Design review of the part shown in the three views and the two pictorial views. Dimensions are in mm from the part's minimum x, y and z. A direction names the side the tool comes from. Round coordinates to 2 decimals unless told otherwise and drop trailing zeros. Loops run counter-clockwise (first coordinate to the right, second up) from the corner with the lowest first, then second, coordinate; pieces in that order, holes last. Notation, with made-up numbers: M 0,-25.75 L 27,-25.75 A16 ccw 27,-6.75 Z; hole C -36,-34 d7. An arc over 180 degrees is marked long. Return JSON: item names as keys, results as strings. Group by question number.
Q1. Consider section D-D (x = 104.5). State the section outline as (y, z) points.
Q2. Consider section B-B (y = 57.15). State the section outline as (x, z) points, and give its area (3 significant figures).
Q3. To check wall thickness, follow line 1 along Y through (x, z) = (57.15, 96.75); line 2 along Z through (x, y) = (24, 40.5). State the ranges of each line that lie inside material, in increasing order.
Q4. Clearance check with flat-ended pins moving along their axes: pin 1 Ø2.5 at (y, z) = (4.5, 4) entering from +X (1 decimal); pin 2 Ø2 at (x, z) = (29, 87.5) entering from -Y; pin 3 Ø5.5 at (x, y) = (57.5, 5) entering from -Z; pin 4 Ø1.5 at (x, y) = (95, 102) entering from -Z. State where each tip first meets the part, or that it passes through.
Q5. Draft analysis for pull direction X (two halves, no side actions). For the marked faces 1 and 2, state which applies: pulls with the +X half, pulls with the -X half, needs draft (parallel to the pull), parting line crosses it, or undercut.
Q6. Consider section A-A (x = 57.15). State the section outline as (y, z) points, and give its area (3 significant figures).
Q7. Consider section C-C (z = 28.5). State the section outline as (x, y) points.
Q8. For the marked faces 3, 4 and 5, list the 3-axis set-ups (+Z, -Z, +X, -X, +Y, -Y) from which the entire face can be reached by the end or side of a thin tool; tool diameter is ignored.
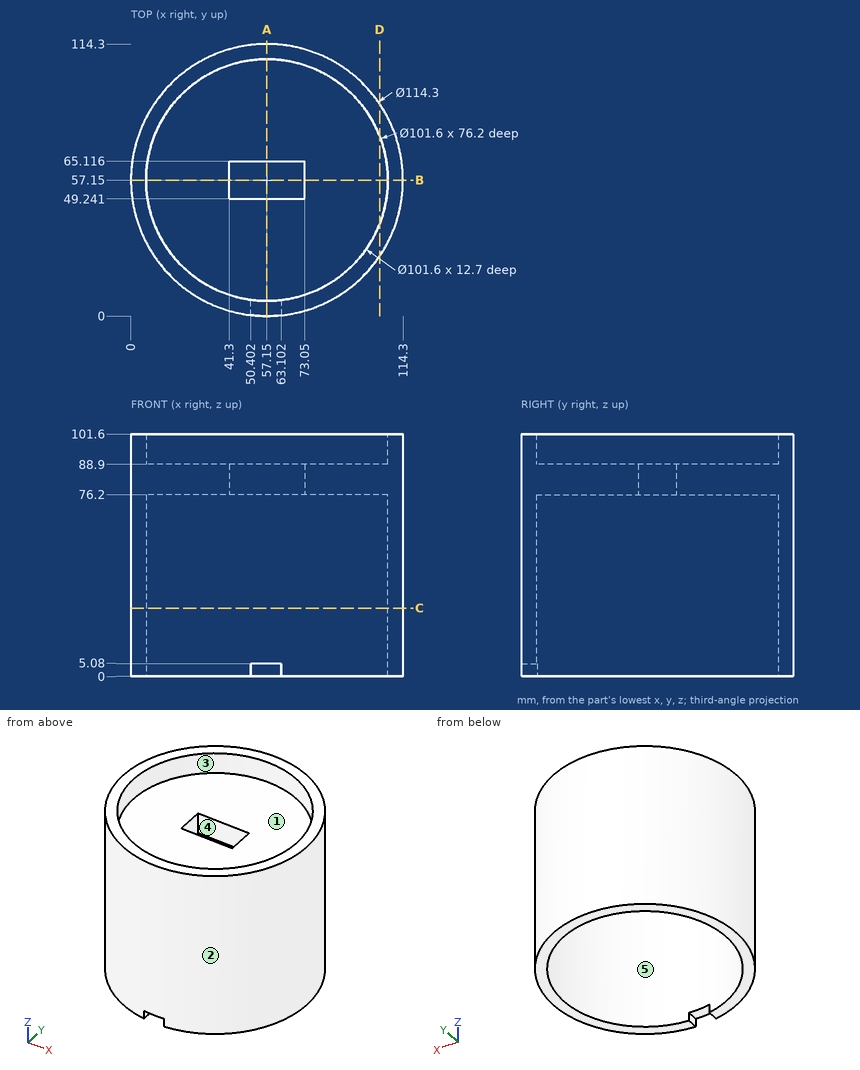
Values:
{
 "1": {"outline": "M 25.15,0 L 38.75,0 L 38.75,76.2 L 75.55,76.2 L 75.55,0 L 89.15,0 L 89.15,101.6 L 75.55,101.6 L 75.55,88.9 L 38.75,88.9 L 38.75,101.6 L 25.15,101.6 Z"},
 "2": {"outline": "M 0,0 L 6.35,0 L 6.35,76.2 L 41.3,76.2 L 41.3,88.9 L 6.35,88.9 L 6.35,101.6 L 0,101.6 Z; M 73.05,76.2 L 107.95,76.2 L 107.95,0 L 114.3,0 L 114.3,101.6 L 107.95,101.6 L 107.95,88.9 L 73.05,88.9 Z", "area": "2,180 mm2"},
 "3": {"line 1": "y = 0 to 6.35, 107.95 to 114.3", "line 2": "z = 76.2 to 88.9"},
 "4": {"pin 1": "stops at x = 82.1", "pin 2": "stops at y = 6.86", "pin 3": "stops at z = 5.08", "pin 4": "passes through"},
 "5": {"face 1": "undercut", "face 2": "parting line crosses it"},
 "6": {"outline": "M 0,5.08 L 6.35,5.08 L 6.35,76.2 L 49.24,76.2 L 49.24,88.9 L 6.35,88.9 L 6.35,101.6 L 0,101.6 Z; M 65.12,76.2 L 107.95,76.2 L 107.95,0 L 114.3,0 L 114.3,101.6 L 107.95,101.6 L 107.95,88.9 L 65.12,88.9 Z", "area": "2,350 mm2"},
 "7": {"outline": "C 57.15,57.15 d114.3; hole C 57.15,57.15 d101.6"},
 "8": {"face 3": "+Z", "face 4": "+Z, -Z", "face 5": "-Z"}
}
